The listing builds one solid part. Answer for the finished solid, in the listing's coordinates (mm). Face numbers are marked on the shaded views. A direction names the side the tool comes from. Round coordinates to 2 decimals unless told otherwise and drop trailing zeros. Write each loop counter-clockwise with the first axis right and the second up, starting at its lowest first coordinate (ties: lowest second). Pieces come first, ordered by that corner, then holes.
Item 1: Each of these flat-tipped pins is pushed along its axis until it touches: pin 1 (8.5 mm diameter, centred on x = 5.5, y = 28, fed in from +Z); pin 2 (8 mm diameter, centred on x = -19, z = 6.5, fed in from +Y); pin 3 (20.5 mm diameter, centred on x = -8, y = -7, fed in from +Z). Where does it stop, or does it pass through?
Item 2: Find section A-A on z = -12.5. Give the vertices of the cut face in (x, y), then the cut area to 3 significant figures.
Item 3: Find the intervals of material crossed by probe 1 along X at (y, z) = (8.5, -3.5); probe 2 along Y at (x, z) = (-6, -3); probe 3 along X at (y, z) = (5, -7), in increasing order.
Item 4: For a pull along Z with two mould halves and no side action, classify the marked faces 4, 5 and 6 as +Z half, -Z half, draft (parallel to the pull), parting line (faces both ways), or undercut.
Item 5: A tool of negligible diameter and unlimited length cuts with its end or side. For the marked faces 1, 2 and 3, from which of +Z, -Z, +X, -X, +Y, -Y can it reach the whole face along a straight path? Write none if from no direction.
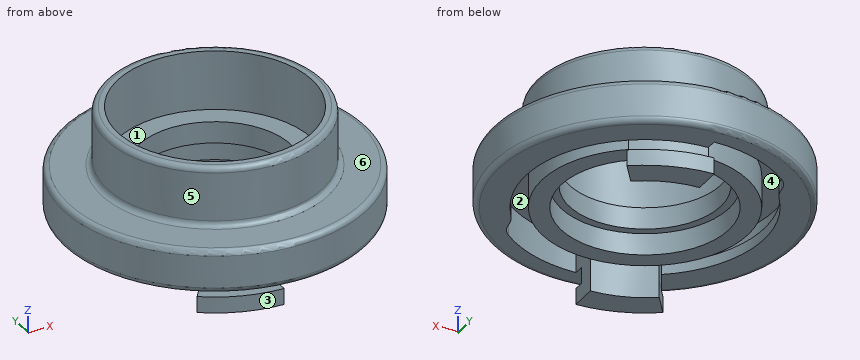
```python
from build123d import *

# Parameters (mm, degrees)
SKETCH1_R           = 25.4
BOSS_EXTRUDE1_DEPTH = 13.97
SKETCH2_R           = 22.86
CUT_EXTRUDE1_DEPTH  = 25.4
SKETCH3_R           = 35.56
BOSS_EXTRUDE2_DEPTH = 10.16
SKETCH4_R           = 17.78
CUT_EXTRUDE2_DEPTH  = 10.16
CUT_EXTRUDE3_DEPTH  = 7.62
CUT_EXTRUDE4_DEPTH  = 5.08
BOSS_EXTRUDE3_START = 3.81
BOSS_EXTRUDE3_DEPTH = 3.81
BOSS_EXTRUDE4_START = 3.81
BOSS_EXTRUDE4_DEPTH = 3.81
FILLET1_R           = 1.27
FILLET2_R           = 1.27
BOSS_EXTRUDE5_START = 3.81
BOSS_EXTRUDE5_DEPTH = 3.81
BOSS_EXTRUDE6_START = 3.81
BOSS_EXTRUDE6_DEPTH = 3.81
SKETCH12_R          = 19.685
SKETCH12_R_2        = 15.494
CUT_EXTRUDE5_DEPTH  = 5.08
CUT_EXTRUDE6_DEPTH  = 7.62
CUT_EXTRUDE7_DEPTH  = 5.08


with BuildPart() as part:
    # Sketch1 → Boss-Extrude1 (new body)
    with BuildSketch(Plane.XY):
        Circle(SKETCH1_R)
    extrude(amount=BOSS_EXTRUDE1_DEPTH)

    # Sketch2 → Cut-Extrude1 (cut)
    with BuildSketch(Plane.XY.offset(13.97)):
        Circle(SKETCH2_R)
    extrude(amount=-CUT_EXTRUDE1_DEPTH, mode=Mode.SUBTRACT)

    # Sketch3 → Boss-Extrude2 (add)
    with BuildSketch(Plane(origin=(0, 0, 0), x_dir=(-1, 0, 0), z_dir=(0, 0, -1))):
        Circle(SKETCH3_R)
    extrude(amount=BOSS_EXTRUDE2_DEPTH)

    # Sketch4 → Cut-Extrude2 (cut)
    with BuildSketch(Plane(origin=(0, 0, -10.16), x_dir=(-1, 0, 0), z_dir=(0, 0, -1))):
        Circle(SKETCH4_R)
    extrude(amount=-CUT_EXTRUDE2_DEPTH, mode=Mode.SUBTRACT)

    # Sketch5 → Cut-Extrude3 (cut)
    with BuildSketch(Plane(origin=(0, 0, -10.16), x_dir=(-1, 0, 0), z_dir=(0, 0, -1))):
        with BuildLine():
            Line((0, 24.13), (0, 30.48))
            ThreePointArc((0, 30.48), (10.414, 28.645750191), (19.574595964, 23.363766667))
            ThreePointArc((19.574595964, 23.363766667), (20.902767484, 21.720232391), (21.5114344, 19.696678812))
            ThreePointArc((21.5114344, 19.696678812), (21.950994255, 17.793379172), (22.86, 16.064370514))
            ThreePointArc((22.86, 16.064370514), (27.516036857, -4.848846843), (15.991836773, -22.9108))
            Line((15.991836773, -22.9108), (13.811131758, -19.7866))
            ThreePointArc((13.811131758, -19.7866), (23.01855293, 7.239), (0, 24.13))
        make_face()
    extrude(amount=-CUT_EXTRUDE3_DEPTH, mode=Mode.SUBTRACT)

    # Sketch7 → Cut-Extrude4 (cut)
    with BuildSketch(Plane(origin=(0, 0, -7.62), x_dir=(-1, 0, 0), z_dir=(0, 0, -1))):
        with BuildLine():
            Line((17.445640116, -24.9936), (15.991836773, -22.9108))
            ThreePointArc((15.991836773, -22.9108), (27.516036857, -4.848846843), (22.86, 16.064370514))
            ThreePointArc((22.86, 16.064370514), (21.950994255, 17.793379172), (21.5114344, 19.696678812))
            ThreePointArc((21.5114344, 19.696678812), (20.902767484, 21.720232391), (19.574595964, 23.363766667))
            ThreePointArc((19.574595964, 23.363766667), (30.450504061, -1.340597786), (17.445640116, -24.9936))
        make_face()
    extrude(amount=-CUT_EXTRUDE4_DEPTH, mode=Mode.SUBTRACT)

    # Sketch8 → Boss-Extrude3 (add)
    with BuildSketch(Plane(origin=(0, 0, -10.16), x_dir=(-1, 0, 0), z_dir=(0, 0, -1)).offset(BOSS_EXTRUDE3_START)):
        with BuildLine():
            Line((0, -27.94), (0, -24.13))
            ThreePointArc((0, -24.13), (7.239, -23.01855293), (13.811131758, -19.7866))
            Line((13.811131758, -19.7866), (15.991836773, -22.9108))
            ThreePointArc((15.991836773, -22.9108), (8.382, -26.653061288), (0, -27.94))
        make_face()
    extrude(amount=-BOSS_EXTRUDE3_DEPTH)

    # Sketch9 → Boss-Extrude4 (add)
    with BuildSketch(Plane(origin=(0, 0, -13.97), x_dir=(-1, 0, 0), z_dir=(0, 0, -1)).offset(BOSS_EXTRUDE4_START)):
        with BuildLine():
            Line((0, -24.13), (0, -30.48))
            ThreePointArc((0, -30.48), (9.144, -29.076066859), (17.445640116, -24.9936))
            Line((17.445640116, -24.9936), (13.811131758, -19.7866))
            ThreePointArc((13.811131758, -19.7866), (7.239, -23.01855293), (0, -24.13))
        make_face()
    extrude(amount=-BOSS_EXTRUDE4_DEPTH)

    # Fillet1
    fillet1_edges = [part.edges().sort_by_distance(p)[0] for p in [
        (35.56, 0, -10.16),
    ]]
    fillet(fillet1_edges, radius=FILLET1_R)

    # Fillet2
    fillet2_edges = [part.edges().sort_by_distance(p)[0] for p in [
        (-25.4, 0, 0),
        (35.56, 0, 0),
        (-25.4, 0, 13.97),
    ]]
    fillet(fillet2_edges, radius=FILLET2_R)

    # Sketch10 → Boss-Extrude5 (add)
    with BuildSketch(Plane(origin=(0, 0, -10.16), x_dir=(-1, 0, 0), z_dir=(0, 0, -1)).offset(BOSS_EXTRUDE5_START)):
        with BuildLine():
            Line((-13.819909091, 19.780470488), (-16.002, 22.90370267))
            ThreePointArc((-16.002, 22.90370267), (-8.387912356, 26.651201217), (0, 27.94))
            Line((0, 27.94), (0, 24.13))
            ThreePointArc((0, 24.13), (-7.244106126, 23.016946505), (-13.819909091, 19.780470488))
        make_face()
    extrude(amount=-BOSS_EXTRUDE5_DEPTH)

    # Sketch11 → Boss-Extrude6 (add)
    with BuildSketch(Plane(origin=(0, 0, -13.97), x_dir=(-1, 0, 0), z_dir=(0, 0, -1)).offset(BOSS_EXTRUDE6_START)):
        with BuildLine():
            Line((-13.819909091, 19.780470488), (-17.486542269, 25.028531737))
            ThreePointArc((-17.486542269, 25.028531737), (-9.166078238, 29.123694325), (0, 30.53205793))
            Line((0, 30.53205793), (0, 24.13))
            ThreePointArc((0, 24.13), (-7.244106126, 23.016946505), (-13.819909091, 19.780470488))
        make_face()
    extrude(amount=-BOSS_EXTRUDE6_DEPTH)

    # Sketch12 → Cut-Extrude5 (cut)
    with BuildSketch(Plane(origin=(0, 0, -10.16), x_dir=(-1, 0, 0), z_dir=(0, 0, -1))):
        Circle(SKETCH12_R)
        Circle(SKETCH12_R_2, mode=Mode.SUBTRACT)
    extrude(amount=-CUT_EXTRUDE5_DEPTH, mode=Mode.SUBTRACT)

    # Sketch13 → Cut-Extrude6 (cut)
    with BuildSketch(Plane(origin=(0, 0, -10.16), x_dir=(-1, 0, 0), z_dir=(0, 0, -1))):
        with BuildLine():
            Line((-16.002, 22.90370267), (-13.819909091, 19.780470488))
            ThreePointArc((-13.819909091, 19.780470488), (-23.016946505, -7.244106126), (0, -24.13))
            Line((0, -24.13), (0, -30.48))
            ThreePointArc((0, -30.48), (-10.414, -28.645750191), (-19.574595964, -23.363766667))
            ThreePointArc((-19.574595964, -23.363766667), (-20.902767484, -21.720232391), (-21.5114344, -19.696678812))
            ThreePointArc((-21.5114344, -19.696678812), (-21.950994255, -17.793379172), (-22.86, -16.064370514))
            ThreePointArc((-22.86, -16.064370514), (-27.51711182, 4.842742724), (-16.002, 22.90370267))
        make_face()
    extrude(amount=-CUT_EXTRUDE6_DEPTH, mode=Mode.SUBTRACT)

    # Sketch15 → Cut-Extrude7 (cut)
    with BuildSketch(Plane(origin=(0, 0, -7.62), x_dir=(-1, 0, 0), z_dir=(0, 0, -1))):
        with BuildLine():
            Line((-17.456727273, 24.985857458), (-16.002, 22.90370267))
            ThreePointArc((-16.002, 22.90370267), (-27.51711182, 4.842742724), (-22.86, -16.064370514))
            ThreePointArc((-22.86, -16.064370514), (-21.950994255, -17.793379172), (-21.5114344, -19.696678812))
            ThreePointArc((-21.5114344, -19.696678812), (-20.902767484, -21.720232391), (-19.574595964, -23.363766667))
            ThreePointArc((-19.574595964, -23.363766667), (-30.450800702, 1.333842788), (-17.456727273, 24.985857458))
        make_face()
    extrude(amount=-CUT_EXTRUDE7_DEPTH, mode=Mode.SUBTRACT)


solid = part.part
```
Check values:
1. pin 1: stops at z = 13.96
1. pin 2: stops at y = 20.5
1. pin 3: stops at z = 0
2. outline: (-15.99, -22.91) arc R27.94 ccw to (0, -27.94) - (0, -24.13) arc R24.13 cw to (-13.81, -19.79) - close; (0, 24.13) arc R24.13 cw to (13.82, 19.78) - (16, 22.9) arc R27.94 ccw to (0, 27.94) - close
2. area: 121 mm2
3. probe 1: x = -34.53 to -29.27, -22.58 to -15.62, 15.62 to 22.58, 29.27 to 34.53
3. probe 2: y = -35.05 to -16.74, 16.74 to 23.37, 29.88 to 35.05
3. probe 3: x = -35.21 to -30.07, -23.61 to -19.04, 19.04 to 23.61, 30.07 to 35.21
4. face 4: undercut
4. face 5: draft
4. face 6: +Z half
5. face 1: +Z
5. face 2: none
5. face 3: -Z, -X, -Y
